Geometry: final body of the model. Coordinates: model frame, mm. A direction names the side the tool comes from. Give positions to 0.01 mm unless a question says otherwise; leave off trailing zeros. Write each loop counter-clockwise with the first axis right and the second up, starting at its lowest first coordinate (ties: lowest second). Pieces come first, ordered by that corner, then holes.
Q1. Line query: line 1 (Z direction, x = -18.5, y = 0.5); line 2 (X direction, y = 0.7, z = 0); line 3 (X direction, y = 2.4, z = 0). Output: solid intervals per line, ascending.
Q2. Section B-B (z = -7.7). Return the cut outline in (x, y).
Q3. Mould query, pull axis X, two halves, no side actions, for faces 1 (the cylindrical face through (-0.316, 12.014, 12.634)), 2 (the flat face through (0, 0, 1)). Classes: +X half, -X half, draft (parallel to the pull), parting line (faces both ways), or undercut.
Q4. Reachability of faces 3 (the flat face through (19, 6, -3)), 4 (the cylindrical face through (0.316, 12.014, -19.196)), 5 (the cylindrical face through (-5.776, 0.493, 0.391)), 6 (the flat face through (-18, 6, -3)) from +Z, -Z, +X, -X, +Y, -Y: full face, straight path, thin tool, end or side. Return the list, or none.
Q5. Section C-C (y = 8.5). Return the cut outline in (x, z), plus the area to 3 significant figures.
Q6. Section A-A (x = 18.5). Return the cut outline in (y, z).
Q7. Section D-D (z = 13.5). Return the cut outline in (x, y).
Q8. Pin query (flat end, axial travel): pin 1 Ø3 at (x, z) = (19.5, 0.5) entering from +Y; pin 2 Ø5 at (x, z) = (8.75, 0) entering from +Y; pin 3 Ø5.5 at (y, z) = (10, -3.5) entering from +X; pin 4 Ø1.8 at (x, z) = (2.7, 10.73) entering from -Y. Return the tip coordinate at first contact, or that it passes through.
from build123d import *

# Parameters (mm, degrees)
SKETCH_1_W          = 27
SKETCH_1_H          = 36
SKETCH_1_R          = 6.75
SKETCH_1_R_2        = 1.5
SKETCH_1_R_3        = 1.25
EXTRUDE_1_DEPTH     = 3
SKETCH_4_W          = 10
SKETCH_4_H          = 6
EXTRUDE_3_DEPTH     = 36
SKETCH_6_R          = 3
CUT_EXTRUDE_3_DEPTH = 1
EXTRUDE_4_OUTLINE_W = 27
EXTRUDE_4_OUTLINE_H = 36
EXTRUDE_4_DEPTH     = 10
CUT_EXTRUDE_START   = 10
CUT_EXTRUDE_5_DEPTH = 2
SKETCH_13_R         = 2
CUT_EXTRUDE_6_DEPTH = 10


# Read off the part's stored shape, not the designer's step: 凸台-拉伸4
with BuildPart() as part:
    # 草图1 → 凸台-拉伸1 (new body)
    with BuildSketch(Plane(origin=(0, 0, 0), x_dir=(1, 0, 0), z_dir=(0, 1, 0))):
        with Locations((0, 2.267700118)):
            Rectangle(SKETCH_1_W, SKETCH_1_H)
        with Locations(Location((0, 7.7, 0), (0, 0, 270))):
            Circle(SKETCH_1_R, mode=Mode.SUBTRACT)
        with Locations(Location((0, -4.3, 0), (0, 0, 270))):
            Circle(SKETCH_1_R_2, mode=Mode.SUBTRACT)
        with Locations(Location((-8.75, 0, 0), (0, 0, 90))):
            Circle(SKETCH_1_R_3, mode=Mode.SUBTRACT)
        with Locations(Location((-2.7, -10.732299882, 0), (0, 0, 90))):
            Circle(SKETCH_1_R_2, mode=Mode.SUBTRACT)
        with Locations(Location((8.75, 0, 0), (0, 0, 270))):
            Circle(SKETCH_1_R_3, mode=Mode.SUBTRACT)
        with Locations(Location((2.7, -10.732299882, 0), (0, 0, 270))):
            Circle(SKETCH_1_R_2, mode=Mode.SUBTRACT)
    extrude(amount=EXTRUDE_1_DEPTH)

    # 草图4 → 凸台-拉伸3 (add)
    with BuildSketch(Plane(origin=(0, 0, -20.267700118), x_dir=(-1, 0, 0), z_dir=(0, 0, -1))):
        with Locations((-18.5, 3)):
            Rectangle(SKETCH_4_W, SKETCH_4_H)
        with Locations((18.5, 3)):
            Rectangle(SKETCH_4_W, SKETCH_4_H)
    extrude(amount=-EXTRUDE_3_DEPTH)

    # 草图6 → 切除-拉伸3 (cut)
    with BuildSketch(Plane.XZ):
        with Locations(Location((-8.75, 0, 0), (0, 0, 270))):
            Circle(SKETCH_6_R)
        with Locations(Location((8.75, 0, 0), (0, 0, 270))):
            Circle(SKETCH_6_R)
    extrude(amount=-CUT_EXTRUDE_3_DEPTH, mode=Mode.SUBTRACT)

    # 凸台-拉伸4 outline → 凸台-拉伸4 (add)
    with BuildSketch(Plane(origin=(0, 3, 0), x_dir=(1, 0, 0), z_dir=(0, 1, 0))):
        with Locations((0, 2.267700118)):
            Rectangle(EXTRUDE_4_OUTLINE_W, EXTRUDE_4_OUTLINE_H)
        with BuildLine():
            ThreePointArc((-1.435964828, -11.539898225), (-3.106363606, -12.176207296), (-4.199704154, -10.762089989))
            ThreePointArc((-4.199704154, -10.762089989), (-9.817841219, -4.861453177), (-9.52470472, 3.280724041))
            ThreePointArc((-9.52470472, 3.280724041), (0, 18.2), (9.52470472, 3.280724041))
            ThreePointArc((9.52470472, 3.280724041), (9.817841219, -4.861453177), (4.199704154, -10.762089989))
            ThreePointArc((4.199704154, -10.762089989), (3.106363606, -12.176207296), (1.435964828, -11.539898225))
            ThreePointArc((1.435964828, -11.539898225), (0, -11.638551918), (-1.435964828, -11.539898225))
        make_face(mode=Mode.SUBTRACT)
    extrude(amount=EXTRUDE_4_DEPTH)

    # 草图9 → 切除-拉伸5 (cut)
    with BuildSketch(Plane(origin=(0, 3, 0), x_dir=(1, 0, 0), z_dir=(0, 1, 0)).offset(CUT_EXTRUDE_START)):
        with BuildLine():
            ThreePointArc((10.616967552, 3.280724041), (0, 19.2), (-10.616967552, 3.280724041))
            ThreePointArc((-10.616967552, 3.280724041), (0, -12.638551918), (10.616967552, 3.280724041))
        make_face()
    extrude(amount=-CUT_EXTRUDE_5_DEPTH, mode=Mode.SUBTRACT)

    # 草图13 → 切除-拉伸6 (cut)
    with BuildSketch(Plane(origin=(0, 6, 0), x_dir=(1, 0, 0), z_dir=(0, 1, 0))):
        with Locations(Location((-18.5, 14.267700118, 0), (0, 0, 180))):
            Circle(SKETCH_13_R)
        with Locations(Location((-18.5, -9.732299882, 0), (0, 0, 180))):
            Circle(SKETCH_13_R)
        with Locations(Location((18.5, -9.732299882, 0), (0, 0, 90))):
            Circle(SKETCH_13_R)
        with Locations(Location((18.5, 14.267700118, 0), (0, 0, 90))):
            Circle(SKETCH_13_R)
    extrude(amount=-CUT_EXTRUDE_6_DEPTH, mode=Mode.SUBTRACT)


solid = part.part
Computed:
1. line 1: z = -20.27 to -16.27, -12.27 to 7.73, 11.73 to 15.73
1. line 2: x = -23.5 to -11.75, -5.75 to 5.75, 11.75 to 23.5
1. line 3: x = -23.5 to -10, -7.5 to 7.5, 10 to 23.5
2. outline: (-23.5, 0) - (-6.75, 0) - (-6.75, 3) - (-10.5, 3) - (-10.5, 11) - (-11.5, 11) - (-11.5, 13) - (-13.5, 13) - (-13.5, 6) - (-23.5, 6) - close; (6.75, 0) - (23.5, 0) - (23.5, 6) - (13.5, 6) - (13.5, 13) - (11.5, 13) - (11.5, 11) - (10.5, 11) - (10.5, 3) - (6.75, 3) - close
3. face 1: undercut
3. face 2: draft
4. face 3: +Z, -Z, +X, +Y
4. face 4: +Y
4. face 5: -Y
4. face 6: +Z, -Z, -X, +Y
5. outline: (-13.5, -20.27) - (13.5, -20.27) - (13.5, 15.73) - (-13.5, 15.73) - close; hole (-9.52, -3.28) arc R10.5 ccw (long way) to (9.52, -3.28) arc R10.5 ccw to (4.2, 10.76) arc R1.5 ccw to (1.44, 11.54) arc R10.5 ccw to (-1.44, 11.54) arc R1.5 ccw to (-4.2, 10.76) arc R10.5 ccw to start
5. area: 442 mm2
6. outline: (0, -20.27) - (6, -20.27) - (6, -16.27) - (0, -16.27) - close; (0, -12.27) - (6, -12.27) - (6, 7.73) - (0, 7.73) - close; (0, 11.73) - (6, 11.73) - (6, 15.73) - (0, 15.73) - close
7. outline: (-23.5, 0) - (23.5, 0) - (23.5, 6) - (13.5, 6) - (13.5, 13) - (-13.5, 13) - (-13.5, 6) - (-23.5, 6) - close
8. pin 1: stops at y = 6
8. pin 2: stops at y = 11
8. pin 3: stops at x = 13.5
8. pin 4: passes through
